from build123d import *

# Parameters (mm, degrees)
BOSS_EXTRUDE1_DEPTH     = 18
CUT_EXTRUDE1_DEPTH      = 44.04814257
CUT_EXTRUDE1_DEPTH_BACK = 44.04814257
SKETCH5_R               = 1.5
CUT_EXTRUDE2_DEPTH      = 44.048142727
CUT_EXTRUDE3_START      = -18
CUT_EXTRUDE3_DEPTH      = 18
FILLET1_R               = 2
CUT_EXTRUDE4_DEPTH      = 24.246649109
CUT_EXTRUDE4_DEPTH_BACK = 2.5


# Read off the part's stored shape, not the designer's step: Cut-Extrude3
with BuildPart() as part:
    # Sketch2 → Boss-Extrude1 (new body)
    with BuildSketch(Plane(origin=(0, 0, 0), x_dir=(1, 0, 0), z_dir=(0, 1, 0))):
        with BuildLine():
            Line((12.654745303, 34.768626969), (9.918584156, 27.251086003))
            Line((9.918584156, 27.251086003), (-4.036019928, 28.717773994))
            Line((-4.036019928, 28.717773994), (-5.149404736, 36.639918543))
            ThreePointArc((-5.149404736, 36.639918543), (3.867553141, 36.797310129), (12.654745303, 34.768626969))
        make_face()
    extrude(amount=BOSS_EXTRUDE1_DEPTH)

    # Sketch3 → Cut-Extrude1 (cut, two sides: drawn at the far end of the back side and taken through both)
    with BuildSketch(Plane(origin=(0, 0, 0), x_dir=(0, 0, -1), z_dir=(1, 0, 0)).offset(-CUT_EXTRUDE1_DEPTH_BACK)):
        with BuildLine():
            Line((38, 13.1), (39.768626969, 13.1))
            Line((39.768626969, 13.1), (39.768626969, 4.9))
            Line((39.768626969, 4.9), (38, 4.9))
            ThreePointArc((38, 4.9), (33.9, 9), (38, 13.1))
        make_face()
    extrude(amount=CUT_EXTRUDE1_DEPTH + CUT_EXTRUDE1_DEPTH_BACK, mode=Mode.SUBTRACT)

    # Sketch5 → Cut-Extrude2 (cut, through all)
    with BuildSketch(Plane.XY):
        with Locations((0, 3.1)):
            Circle(SKETCH5_R)
        with Locations((0, 14.9)):
            Circle(SKETCH5_R)
    extrude(amount=-CUT_EXTRUDE2_DEPTH, mode=Mode.SUBTRACT)

    # Cut-Extrude3 outline → Cut-Extrude3 (cut)
    with BuildSketch(Plane(origin=(0, 18, 0), x_dir=(1, 0, 0), z_dir=(0, 1, 0)).offset(CUT_EXTRUDE3_START)):
        with BuildLine():
            ThreePointArc((-5.079818185, 36.144784509), (3.815289276, 36.300049142), (12.483735924, 34.298780407))
            Line((12.483735924, 34.298780407), (12.654745303, 34.768626969))
            ThreePointArc((12.654745303, 34.768626969), (3.867553141, 36.797310129), (-5.149404736, 36.639918543))
            Line((-5.149404736, 36.639918543), (-5.079818185, 36.144784509))
        make_face()
    extrude(amount=CUT_EXTRUDE3_DEPTH, mode=Mode.SUBTRACT)

    # Fillet1
    fillet1_edges = [part.edges().sort_by_distance(p)[0] for p in [
        (11.201159694, 18, -30.774933331),
        (11.201159694, 0, -30.774933331),
        (-4.557919056, 0, -32.431279251),
        (-4.557919056, 18, -32.431279251),
    ]]
    fillet(fillet1_edges, radius=FILLET1_R)

    # Sketch7 → Cut-Extrude4 (cut, two sides: drawn at the far end of the back side and taken through both)
    with BuildSketch(Plane.XY.offset(-28.717773994).offset(-CUT_EXTRUDE4_DEPTH_BACK)):
        Polygon((3.175426481, 14.9), (1.58771324, 17.65), (-1.58771324, 17.65), (-3.175426481, 14.9), (-1.58771324, 12.15), (1.58771324, 12.15), align=None)
        Polygon((3.175426481, 3.1), (1.58771324, 5.85), (-1.58771324, 5.85), (-3.175426481, 3.1), (-1.58771324, 0.35), (1.58771324, 0.35), align=None)
    extrude(amount=CUT_EXTRUDE4_DEPTH + CUT_EXTRUDE4_DEPTH_BACK, mode=Mode.SUBTRACT)


solid = part.part
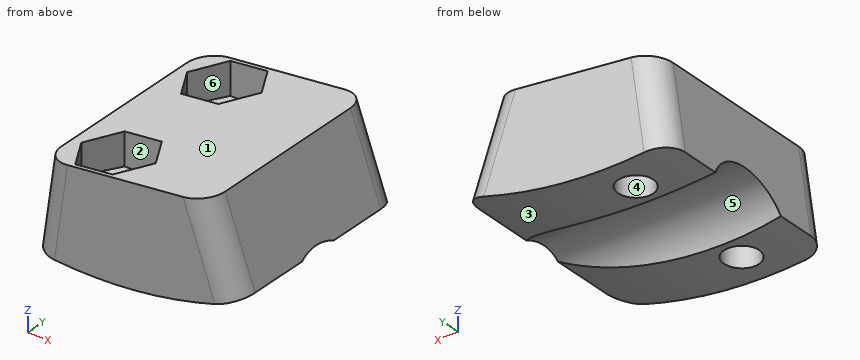
The model under review builds one solid part; all positions refer to its coordinate system, in mm. Face numbers are marked on the shaded views. A direction names the side the tool comes from. Coordinates: 2 decimals unless noted, no trailing zeros. Write each loop counter-clockwise with the first axis right and the second up, starting at its lowest first coordinate (ties: lowest second). Pieces come first, ordered by that corner, then holes. Notation, with made-up numbers: (22.5, -10) - (80.5, -10) arc R24 ccw to (80.5, 4) - close; hole circle Ø8 at (-10, 33). An arc over 180 degrees is marked (long way). Answer as CSV lines item,"result".
(1) Mouldability with a two-part tool opening along X and no side actions: class the marked faces 3, 4, 5 and 6 as pulls with the +X half, pulls with the -X half, needs draft (parallel to the pull), parting line crosses it, or undercut.
Data:
face 3,"parting line crosses it"
face 4,"undercut"
face 5,"needs draft"
face 6,"undercut"
(2) For line 1 along Y through (x, z) = (0, -32.9); line 2 along Y through (x, z) = (0, -35.25); line 3 along Y through (x, z) = (0, -34.85), list the stretches that pass through material, from the lowest coordinate up. Write a range as [from, to].
Data:
line 1,"y = [0, 1.6], [4.6, 13.4], [16.4, 18]"
line 2,"y = [0, 1.6], [4.6, 5.96], [12.04, 13.4], [16.4, 18]"
line 3,"y = [0, 1.6], [4.6, 6.38], [11.62, 13.4], [16.4, 18]"
(3) We need section B-B (x = 0). Give the boundary of the cut face in (y, z), plus the area to 3 significant figures.
Data:
outline,"(0, -36.5) - (1.6, -36.5) - (1.6, -31.22) - (0.35, -31.22) - (0.35, -28.29) - (0, -28.29) - close; (4.6, -36.5) - (5.18, -36.5) arc R4.1 cw to (12.82, -36.5) - (13.4, -36.5) - (13.4, -31.22) - (12.15, -31.22) - (12.15, -28.29) - (5.85, -28.29) - (5.85, -31.22) - (4.6, -31.22) - close; (16.4, -36.5) - (18, -36.5) - (18, -28.29) - (17.65, -28.29) - (17.65, -31.22) - (16.4, -31.22) - close"
area,"69.5 mm2"
(4) Tool access review of the marked faces 1 and 2: name each direction out of +Z, -Z, +X, -X, +Y, -Y from which nothing blocks a thin tool from reaching the whole face with its end or side.
Data:
face 1,"+Z, -X, +Y, -Y"
face 2,"+Z"
(5) We need section C-C (x = 6.25). Give the boundary of the cut face in (y, z), plus the area to 3 significant figures.
Data:
outline,"(0, -35.96) - (5.44, -35.96) arc R4.1 cw to (12.56, -35.96) - (18, -35.96) - (18, -27.64) - (0, -27.64) - close"
area,"139 mm2"
(6) We need section D-D (x = 2.75). Give the boundary of the cut face in (y, z).
Data:
outline,"(0, -36.4) - (5.23, -36.4) arc R4.1 cw to (12.77, -36.4) - (18, -36.4) - (18, -28) - (15.64, -28) - (15.64, -31.22) - (14.16, -31.22) - (14.16, -28) - (3.84, -28) - (3.84, -31.22) - (2.36, -31.22) - (2.36, -28) - (0, -28) - close"
(7) Clearance check with flat-ended pins moving along their axes: pin 1 Ø4 at (x, y) = (9.5, 8) entering from -Z; pin 2 Ø2 at (y, z) = (9.5, -28) entering from +X; pin 3 Ø2 at (x, y) = (7.5, 10.5) entering from -Z; pin 4 Ø5 at (x, z) = (7, -32) entering from -Y. State where each tip first meets the part, or that it passes through.
Data:
pin 1,"stops at z = -35.21"
pin 2,"stops at x = 10.56"
pin 3,"stops at z = -34.75"
pin 4,"stops at y = 0"
(8) We need section A-A (y = 14.25). Give the boundary of the cut face in (x, z).
Data:
outline,"(-5.08, -36.14) arc R36.5 ccw to (-1.35, -36.47) - (-1.35, -31.22) - (-2.8, -31.22) - (-2.8, -28.59) - (-4.04, -28.72) - close; (1.35, -36.47) arc R36.5 ccw to (12.48, -34.3) - (9.92, -27.25) - (2.8, -28) - (2.8, -31.22) - (1.35, -31.22) - close"
